from build123d import *

# Parameters (mm, degrees)
F0_R     = 52
F0_R_2   = 1.5
F1_DEPTH = 5
F3_DEPTH = 2
F4_DEPTH = 2.001


with BuildPart() as f1:
    # F0 (on Top) → F1 (new body)
    with BuildSketch(Plane.XY):
        Circle(F0_R)
        with Locations((0, -42.05)):
            Circle(F0_R_2, mode=Mode.SUBTRACT)
        with Locations((-46.5, 0)):
            Circle(F0_R_2, mode=Mode.SUBTRACT)
        with Locations((46.5, 0)):
            Circle(F0_R_2, mode=Mode.SUBTRACT)
        with Locations((0, 42.05)):
            Circle(F0_R_2, mode=Mode.SUBTRACT)
    extrude(amount=F1_DEPTH)

    # F2 (on Top) → F3 (join)
    with BuildSketch(Plane.XY):
        with BuildLine():
            Line((-24.5919874092, 51.6990972384), (-58, 35.807728358))
            Line((-58, 35.807728358), (-58, 0))
            Line((-58, 0), (-58, -35.807728358))
            Line((-58, -35.807728358), (-24.5919874092, -51.6990972384))
            ThreePointArc((-24.5919874092, -51.6990972384), (0, -57.25), (24.5919874092, -51.6990972384))
            Line((24.5919874092, -51.6990972384), (58, -35.2185990722))
            Line((58, -35.2185990722), (58, 0))
            Line((58, 0), (58, 35.2185990722))
            Line((58, 35.2185990722), (24.5919874092, 51.6990972384))
            ThreePointArc((24.5919874092, 51.6990972384), (0, 57.25), (-24.5919874092, 51.6990972384))
        make_face()
    extrude(amount=F3_DEPTH)

    # F4 (cut, through all): faces of the model
    f4_faces = [f1.faces().sort_by_distance(p)[0] for p in [
        (0, 42.05, 2),
        (46.5, 0, 2),
        (0, -42.05, 2),
        (-46.5, 0, 2),
    ]]
    extrude(f4_faces, amount=-F4_DEPTH, mode=Mode.SUBTRACT)


solid = f1.part
Can you work these out from the model? Positions are in its coordinate system, mm. A direction names the side the tool comes from. Round coordinates to 2 decimals unless told otherwise and drop trailing zeros. Loops run counter-clockwise (first coordinate to the right, second up) from the corner with the lowest first, then second, coordinate; pieces in that order, holes last. Notation, with made-up numbers: (80, 48) - (94, 48) arc R23 cw to (94, 74) - close; hole circle Ø7 at (-7.5, 87.25). An arc over 180 degrees is marked (long way). Write item = value, one per line. Start each with the question number.
(1) If we section it at C-C (y = -42.05): Please give me the cut outline in (x, z), and give its area (3 significant figures).
(2) If we section it at B-B (z = 1): Please give me the cut outline in (x, y), and give its area (3 significant figures).
(3) For P1, Ø10, axis at x = -34, y = -39.5, coming from the -Z side; P2, Ø1, axis at y = -11, z = 4.5, coming from the -X side, each with a flat end and sliding along its axis, tell me the tip position at first contact or that it passes through.
(4) If we section it at D-D (x = 46.5): Please give me the cut outline in (y, z).
(5) If we section it at A-A (x = 0): Please give me the cut outline in (y, z).
(6) If we mould it in two halves opening along X, with no side actions, what happens to faces 1 (the face through (41.53, 43.343, 0.986)), 2 (the face through (45, 0, 3)), 3 (the face through (-1, 1, 0)), 4 (the face through (-0.195, -43.537, 2.535))? For each: released by +X, released by -X, zero draft, split by the parting line, or undercut.
(7) For faces 5 (the face through (0.36, 57.25, 0.99)), 6 (the face through (-41.265, -31.641, 3.479)), which set-ups out of +Z, -Z, +X, -X, +Y, -Y let a thin tool reach every point of the face, with its end or its side?
(8) If I drill on probe 1 along Y at (x, z) = (0, 3.3); probe 2 along Y at (x, z) = (46.5, 1.4); probe 3 along Y at (x, z) = (-20, 3.7), over which ranges is the centre line in solid material (lowest first)? Write a range as [from, to].
Ans:
q1.outline = (-44.88, 0) - (-1.5, 0) - (-1.5, 5) - (-30.59, 5) - (-30.59, 2) - (-44.88, 2) - close; (1.5, 0) - (44.15, 0) - (44.15, 2) - (30.59, 2) - (30.59, 5) - (1.5, 5) - close
q1.area = 347 mm²
q2.outline = (-58, -35.81) - (-24.59, -51.7) arc R57.25 ccw to (24.59, -51.7) - (58, -35.22) - (58, 35.22) - (24.59, 51.7) arc R57.25 ccw to (-24.59, 51.7) - (-58, 35.81) - close; hole circle Ø3 at (-46.5, 0); hole circle Ø3 at (0, -42.05); hole circle Ø3 at (0, 42.05); hole circle Ø3 at (46.5, 0)
q2.area = 11,300 mm²
q3.P1 = 0
q3.P2 = -50.93
q4.outline = (-40.89, 0) - (-1.5, 0) - (-1.5, 5) - (-23.28, 5) - (-23.28, 2) - (-40.89, 2) - close; (1.5, 0) - (40.89, 0) - (40.89, 2) - (23.28, 2) - (23.28, 5) - (1.5, 5) - close
q5.outline = (-57.25, 0) - (-43.55, 0) - (-43.55, 5) - (-52, 5) - (-52, 2) - (-57.25, 2) - close; (-40.55, 0) - (40.55, 0) - (40.55, 5) - (-40.55, 5) - close; (43.55, 0) - (57.25, 0) - (57.25, 2) - (52, 2) - (52, 5) - (43.55, 5) - close
q6.face_1 = released by +X
q6.face_2 = undercut
q6.face_3 = zero draft
q6.face_4 = undercut
q7.face_5 = +Z, -Z, +Y
q7.face_6 = +Z
q8.probe_1 = [-52, -43.55], [-40.55, 40.55], [43.55, 52]
q8.probe_2 = [-40.89, -1.5], [1.5, 40.89]
q8.probe_3 = [-48, 48]
